```python
from build123d import *

# Parameters (mm, degrees)
CHAMFER1_SIZE = 1


with BuildPart() as part:
    # Sketch1 → Revolve1 (revolve)
    with BuildSketch(Plane.XY):
        with BuildLine():
            Line((27.5, 0), (29.936442743, 0))
            ThreePointArc((29.936442743, 0), (32.167974855, 0.680321637), (34.399506968, 0))
            Line((34.399506968, 0), (39, 0))
            Line((39, 0), (39, 4.8))
            Line((39, 4.8), (27.5, 4.8))
            Line((27.5, 4.8), (27.5, 0))
        make_face()
    revolve(axis=Axis((0, 0, 0), (0, 1, 0)))

    # Chamfer1
    chamfer1_edges = [part.edges().sort_by_distance(p)[0] for p in [
        (-39, 4.8, 0),
    ]]
    chamfer(chamfer1_edges, length=CHAMFER1_SIZE)


solid = part.part
```
Source: CAD feature listing. Evaluate the final solid. Frame: model axes, mm. Coordinates: 2 decimals unless noted, no trailing zeros. Loops run counter-clockwise (first coordinate to the right, second up) from the corner with the lowest first, then second, coordinate; pieces in that order, holes last. Notation, with made-up numbers: M 9,40 L 39,40 A16 cw 39,48 Z; hole C 40,-2 d7. An arc over 180 degrees is marked long. Use a Markdown table: item, result. Add a question column.
Q1. Material intervals for L1, parallel to Z at x = 0, y = 2.6; L2, parallel to X at y = 3.15, z = -14, sorted ascending.
Q2. Section query B-B, the plane z = 0. Return loops of the section in (x, y), and give its area (3 significant figures).
Q3. First-contact query: pin 1 (5 mm diameter, centred on x = 3, z = 30.5, fed in from -Y); pin 2 (1.5 mm diameter, centred on y = 4, z = -12.5, fed in from -X); pin 3 (1 mm diameter, centred on x = -10.5, y = 3, fed in from -Z). Flat tips, straight axial feed; report the tip coordinate or a pass-through.
Q4. Section query C-C, the plane y = 3. Return loops of the section in (x, z).
Q5. Draft query along Z for faces 1 (the cylindrical face through (-5.961, 2.366, 26.846)), 2 (the cylindrical face through (-5.077, 1.927, -38.668)), 3 (the flat face through (25.2, 4.8, -11.4)). Return one class per face: pulls with the +Z half, pulls with the -Z half, needs draft (parallel to the pull), parting line crosses it, or undercut.
Q6. Section query A-A, the plane x = 0. Return loops of the section in (y, z).
Result:
| question | item | result |
|---|---|---|
| 1 | L1 | z = -39 to -27.5, 27.5 to 39 |
| 1 | L2 | x = -36.4 to -23.67, 23.67 to 36.4 |
| 2 | outline | M -39,0 L -34.4,0 A4 cw -29.94,0 L -27.5,0 L -27.5,4.8 L -38,4.8 L -39,3.8 Z; M 27.5,0 L 29.94,0 A4 cw 34.4,0 L 39,0 L 39,3.8 L 38,4.8 L 27.5,4.8 Z |
| 2 | area | 105 mm2 |
| 3 | pin 1 | stops at y = 0 |
| 3 | pin 2 | stops at x = -37.18 |
| 3 | pin 3 | stops at z = -37.7 |
| 4 | outline | C 0,0 d78; hole C 0,0 d55 |
| 5 | face 1 | undercut |
| 5 | face 2 | parting line crosses it |
| 5 | face 3 | needs draft |
| 6 | outline | M 0,-39 L 3.8,-39 L 4.8,-38 L 4.8,-27.5 L 0,-27.5 L 0,-29.94 A4 cw 0,-34.4 Z; M 0,27.5 L 4.8,27.5 L 4.8,38 L 3.8,39 L 0,39 L 0,34.4 A4 cw 0,29.94 Z |
